Autodesk Fusion 360 part; units mm, degrees
sketch "Sketch1" plane through (0, 0, 0) normal (0, 0, 1) x (1, 0, 0)
  circle A0 centre (0, 0) radius 1.5
  circle A1 centre (0, 0) radius 16.9
  circle A2 centre (0, 0) radius 14.6
  line L0 (0, 0) -> (25.4189, 0) construction
  line L1 (-6.75, -9.6177) -> (-6.75, 9.6177) construction
  line L2 (6.75, 9.6177) -> (6.75, -10.6368) construction
  line L3 (-6.75, 9.6177) -> (-6.75, 5)
  line L4 (6.75, 5) -> (6.75, 9.6177)
  line L5 (-6.75, -9.6177) -> (-6.75, -5)
  line L6 (6.75, -9.6177) -> (6.75, -5)
  line L7 (-10.6331, 5) -> (-13.7171, 5)
  line L8 (-13.7171, -5) -> (-10.6331, -5)
  arc A3 (-5, -10.6331) -> (5, -10.6331) centre (0, 0) ccw
  line L9 (13.7171, 5) -> (10.6331, 5)
  line L10 (10.6331, -5) -> (13.7171, -5)
  arc A4 (6.75, -9.6177) -> (10.6331, -5) centre (0, 0) ccw
  arc A5 (-6.75, 9.6177) -> (-10.6331, 5) centre (0, 0) ccw
  arc A6 (-10.6331, -5) -> (-6.75, -9.6177) centre (0, 0) ccw
  line L11 (-13.3404, 6) -> (-13.3404, -6) construction
  line L12 (13.3404, -6) -> (13.3404, 6) construction
  line L13 (-11.0797, 6) -> (-13.3404, 6)
  line L14 (11.0797, 6) -> (13.3404, 6)
  line L15 (13.3101, -6) -> (11.0797, -6)
  line L16 (-13.3101, -6) -> (-11.0797, -6)
  line L17 (-13.3404, -6) -> (-11.0797, -6) construction
  line L18 (-11.0797, 6) -> (-13.3404, 6) construction
  arc A7 (11.0797, 6) -> (-11.0797, 6) centre (0, 0) ccw
  line L19 (13.3404, 6) -> (11.0797, 6) construction
  line L20 (10.1026, 6) -> (-10.1026, 6) construction
  arc A8 (-11.0797, -6) -> (11.0797, -6) centre (0, 0) ccw
  line L21 (-10.1026, -6) -> (10.1026, -6) construction
  line L22 (11.0797, -6) -> (13.3404, -6) construction
  arc A9 (10.6331, 5) -> (6.75, 9.6177) centre (0, 0) ccw
  arc A10 (5, 10.6331) -> (-5, 10.6331) centre (0, 0) ccw
  line L23 (-5, -10.6368) -> (-5, -5)
  line L24 (-5, 5) -> (-5, 10.6368)
  line L25 (5, 10.6368) -> (5, 5)
  line L26 (5, -5) -> (5, -10.6368)
  line L27 (-5, 5) -> (-5, 2.5)
  line L28 (-5, 2.5) -> (-6.75, 2.5)
  line L29 (-6.75, 2.5) -> (-6.75, 5)
  line L30 (-5, -5) -> (-5, -2.5)
  line L31 (-5, -2.5) -> (-6.75, -2.5)
  line L32 (-6.75, -2.5) -> (-6.75, -5)
  line L33 (6.75, -5) -> (6.75, -2.5)
  line L34 (6.75, -2.5) -> (5, -2.5)
  line L35 (5, -2.5) -> (5, -5)
  line L36 (6.75, 5) -> (6.75, 2.5)
  line L37 (6.75, 2.5) -> (5, 2.5)
  line L38 (5, 2.5) -> (5, 5)
  line L39 (1.5, -11.75) -> (-1.5, -11.75) construction
  line L40 (-1.5, -11.75) -> (-1.5, 11.75) construction
  line L41 (-1.5, 11.75) -> (1.5, 11.75) construction
  line L42 (1.5, 11.75) -> (1.5, -11.75) construction
  line L43 (1.5, -11.75) -> (-1.5, 11.75) construction
  line L44 (-1.5, -11.75) -> (1.5, 11.75) construction
  arc A11 (-0.7598, -5.9517) -> (0.7598, -5.9517) centre (0, 0) ccw
  line L45 (-0.7598, -5.9517) -> (-1.4879, -11.6554)
  line L46 (0.7598, -5.9517) -> (1.5, -11.75)
  arc A12 (0.7598, 5.9517) -> (-0.7598, 5.9517) centre (0, 0) ccw
  line L47 (-0.7598, 5.9517) -> (-1.4879, 11.6554)
  line L48 (1.5, 11.6539) -> (0.7598, 5.9517)
  line L49 (0, 0) -> (0, 17.8654) construction
  line L50 (0, 0) -> (0, -17.7378) construction
  arc A13 (1.9907, -14.4637) -> (-1.9907, -14.4637) centre (0, -18.52) ccw
  arc A14 (-2.0011, 14.4622) -> (2.0011, 14.4622) centre (0, 18.5154) ccw
  dimension "d1" = 3
  dimension "d2" = 23.5
  dimension "d4" = 33.8
  dimension "d5" = 29.2
  dimension "d10" = 12
  dimension "d11" = 2.5
  dimension "d12" = 2.5
  dimension "d13" = 2.5
  dimension "d14" = 2.5
  dimension "d15" = 3
  dimension "d16" = 23.5
  dimension "d18" = 6
  dimension "d19" = 6
extrude "Extrude1" add sketch "Sketch1" along normal blind 2 contours A2 L3 L4 L5 L6 L7 L8 A3 L9 L10 A4 A5 A6 A9 A10 L23 L24 L25 L26 L27 L28 L29 L30 L31 L32 L33 L34 L35 L36 L37 L38 A11 L45 L46 A12 L47 L48
extrude "Extrude2" add sketch "Sketch1" along normal blind 3 contours A10 A12 L47 L48
chamfer "Chamfer1" distance 5.75 distance2 1 1 edges at (0, 6, 3) measured on face at (0.9217, 9.7816, 3)
extrude "Extrude3" add sketch "Sketch1" along normal blind 3 contours A3 A11 L45 L46
chamfer "Chamfer2" distance 5.75 distance2 1 1 edges at (0, -6, 3) measured on face at (-0.7463, -9.7965, 3)
extrude "Extrude4" add sketch "Sketch1" along normal blind 5 contours A1 | A2 A14 | A2 A13
extrude "Extrude5" add sketch "Sketch1" along normal blind 5 contours A2 L13 L14 A7 A14 | A2 L15 L16 A8 A13
extrude "Extrude6" cut sketch "Sketch1" along normal blind 4 contours A2 L13 L14 A7 A14 | A2 L15 L16 A8 A13
fillet "Fillet1" radius 0.5 1 edges at (-15.7563, -6.1113, 5)
component "Holder" placed x (1, 0, 0) y (0, 1, 0) z (0, 0, 1) at (0, 0, 0)
component "stem" placed x (1, 0, 0) y (0, 1, 0) z (0, 0, 1) at (0, 0, 0)
Source: CAD feature listing. Evaluate the final solid. Frame: model axes, mm. A direction names the side the tool comes from. Round coordinates to 2 decimals unless told otherwise and drop trailing zeros. Order: outer loops, then holes, each group sorted by start corner. A loop starts at its lowest first (then second) coordinate and runs counter-clockwise, first axis right, second up. Notation, with made-up numbers: (-27, 53) -> (-4, 53) arc R25 ccw to (-4, 69) -> close; hole circle Ø11 at (-7, -1). An arc over 180 degrees is marked (long way). Answer as CSV lines item,"result".
Item 1: Pull-direction query (X, two-part tool) for faces 3 (the face through (-12, 5, 1)), 4 (the face through (-0.016, -8.915, 2.507)); classes: pulls with the +X half, pulls with the -X half, needs draft (parallel to the pull), parting line crosses it, or undercut.
A:
face 3,"undercut"
face 4,"undercut"
Item 2: Reachability of faces 1 (the face through (0.021, 8.915, 2.507)), 2 (the face through (-12.2, 6, 4.5)) from +Z, -Z, +X, -X, +Y, -Y: full face, straight path, thin tool, end or side. Return the list, or none.
A:
face 1,"+Z"
face 2,"+Z, -Z"
Item 3: Section D-D, the plane z = 3.6. Return loops of the section in (x, y).
A:
outline,"circle Ø33.8 at (0, 0); hole (-2, 14.46) arc R14.6 ccw to (-1.99, -14.46) arc R4.52 cw to (1.99, -14.46) arc R14.6 ccw to (2, 14.46) arc R4.52 cw to start"
Item 4: Pin query (flat end, axial travel): pin 1 Ø2 at (x, z) = (-12, 1) entering from -Y; pin 2 Ø1.6 at (y, z) = (6, 1) entering from -X; pin 3 Ø2 at (y, z) = (-6, 1) entering from +X; pin 4 Ø1.8 at (x, y) = (0, 0) entering from +Z. Return the tip coordinate at first contact, or that it passes through.
A:
pin 1,"y = -12.83"
pin 2,"x = -16.08"
pin 3,"x = 16.14"
pin 4,"through"
Item 5: Section B-B, the plane x = 0. Count the separate pieces of the cut face and the enclosed holes in it, plus the area to 3 significant figures.
A:
separate pieces,"4"
enclosed holes,"0"
area,"78.5 mm²"
Item 6: Line query: L1, parallel to Y at x = 0, z = 1.4; L2, parallel to Y at x = 3, z = 1.75; L3, parallel to Y at x = -8.5, z = 1. Output: solid intervals per line, ascending.
A:
L1,"-16.9 to -14, -11.75 to -1.5, 1.5 to 11.75, 14 to 16.9"
L2,"-16.63 to -14.29, -11.36 to 11.36, 14.29 to 16.63"
L3,"-14.61 to -11.87, -8.11 to 8.11, 11.87 to 14.61"
Item 7: Section A-A, the plane y = 0. Return loops of the section in (x, z).
A:
outline,"(-16.9, 0) -> (-1.5, 0) -> (-1.5, 2) -> (-14.6, 2) -> (-14.6, 5) -> (-16.4, 5) arc R0.5 ccw to (-16.9, 4.5) -> close; (1.5, 0) -> (16.9, 0) -> (16.9, 4.5) arc R0.5 ccw to (16.4, 5) -> (14.6, 5) -> (14.6, 2) -> (1.5, 2) -> close"
